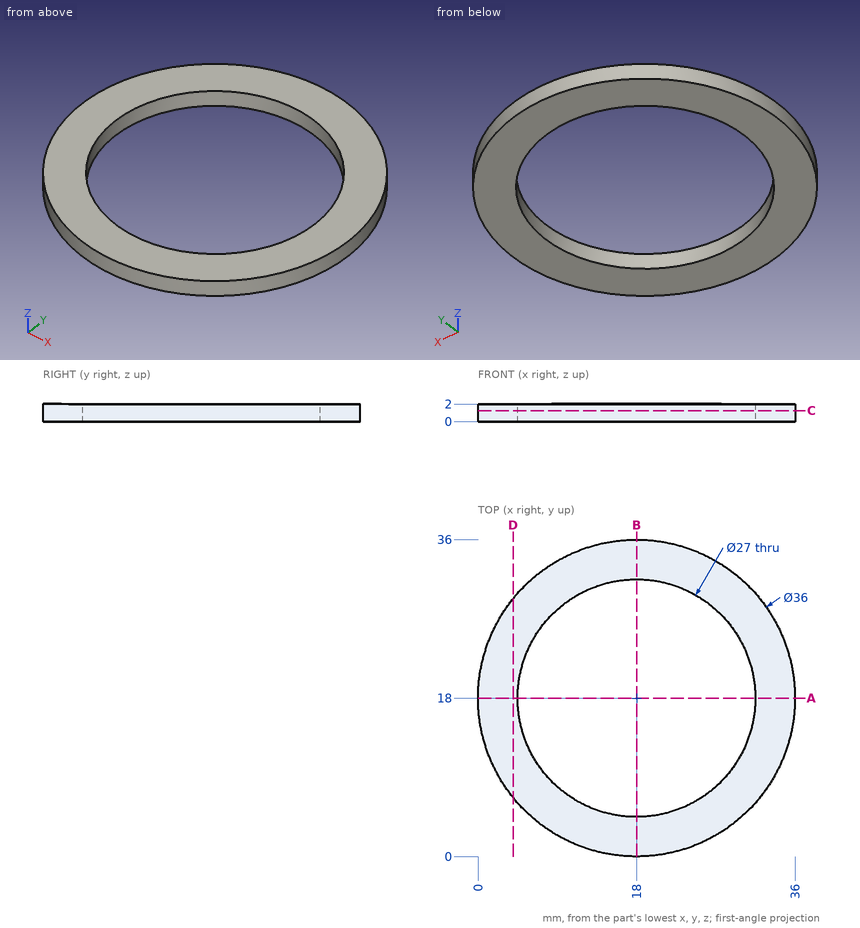
Geometry: see drawing. Coordinates: mm, zero at the bounding-box minimum. Coordinates: 2 decimals unless noted, no trailing zeros. Order: outer loops, then holes, each group sorted by start corner. A loop starts at its lowest first (then second) coordinate and runs counter-clockwise, first axis right, second up. Notation, with made-up numbers: (-29, 14.25) - (9, 14.25) arc R12 cw to (9, 29.25) - close; hole circle Ø9 at (36, 13.5). An arc over 180 degrees is marked (long way). Return JSON: item names as keys, results as strings.
Q1. Cut plane C-C (z = 1.25). Return loops of the section in (x, y).
The answers:
{"outline": "circle Ø36 at (18, 18); hole circle Ø27 at (18, 18)"}
Q2. Ray query, probe 1 along X at (y, z) = (18, 1.4); probe 2 along X at (y, z) = (28.5, 0.55). Return the intervals inside material, ascending.
The answers:
{"probe 1": "x = 0 to 4.5, 31.5 to 36", "probe 2": "x = 3.38 to 9.51, 26.49 to 32.62"}
Q3. First-contact query: pin 1 (1 mm diameter, centred on y = 31, z = 1, fed in from +X); pin 2 (4 mm diameter, centred on x = 11.5, y = 7, fed in from +Z). Flat tips, straight axial feed; report the tip coordinate or a pass-through.
The answers:
{"pin 1": "stops at x = 30.95", "pin 2": "stops at z = 2"}
Q4. Cut plane A-A (y = 18). Return loops of the section in (x, z), then the cut area to 3 significant figures.
The answers:
{"outline": "(0, 0) - (4.5, 0) - (4.5, 2) - (0, 2) - close; (31.5, 0) - (36, 0) - (36, 2) - (31.5, 2) - close", "area": "18.0 mm2"}
Q5. Cut plane D-D (x = 4). Return loops of the section in (y, z), then the cut area to 3 significant figures.
The answers:
{"outline": "(6.69, 0) - (29.31, 0) - (29.31, 2) - (6.69, 2) - close", "area": "45.3 mm2"}
